Autodesk Inventor part; units mm, degrees
ref_plane "YZ Plane" through (0, 0, 0) normal (1, 0, 0) x (0, 1, 0)
ref_plane "XZ Plane" through (0, 0, 0) normal (0, 1, 0) x (-1, 0, 0)
ref_plane "XY Plane" through (0, 0, 0) normal (0, 0, 1) x (1, 0, 0)
sketch "Sketch1" plane through (0, 0, 0) normal (0, 0, 1) x (1, 0, 0)
  line L0 (-18.2, 27.5) -> (18.2, 27.5)
  line L1 (18.2, 27.5) -> (18.2, -27.5)
  line L2 (18.2, -27.5) -> (-18.2, -27.5)
  line L3 (-18.2, -27.5) -> (-18.2, 27.5)
  line L4 (0, -38.5) -> (0, 38.5)
  line L5 (-25.48, 0) -> (25.48, 0)
  circle A0 centre (-12.2, 21.5) radius 3
  circle A1 centre (-12.2, 21.5) radius 6 construction
  circle A2 centre (-12.2, -3.5) radius 3
  line L6 (-12.2, 27.5) -> (-12.2, -3.5) construction
  circle A3 centre (12.2, 21.5) radius 3
  circle A4 centre (12.2, -3.5) radius 3
  point P0 (0, 0)
  point P1 (0, 27.5)
  point P2 (-18.2, 0)
  dimension "d0" = 36.4
  dimension "d1" = 55
  dimension "d2" = 6
  dimension "d3" = 3
  dimension "d34" = 25
extrude "Extrusion1" add sketch "Sketch1" along normal blind 10
sketch "Sketch4" plane through (18.2, -27.5, 0) normal (1, 0, 0) x (0, 0, -1)
  circle A0 centre (-5, 17.5) radius 3 construction
  line L0 (-10, 55) -> (-10, 0)
  line L1 (-10, 27.5) -> (0, 27.5) construction
  line L2 (0, 55) -> (0, 0)
  circle A1 centre (-5, 37.5) radius 3
  line L3 (0, 0) -> (-10, 0)
  line L4 (-5, 0) -> (-5, 55) construction
  line L5 (0, 55) -> (-10, 55)
  circle A2 centre (-5, 17.5) radius 3.1
  dimension "d20" = 6
  dimension "d21" = 20
  dimension "d24" = 6.2
extrude "Extrusion4" cut sketch "Sketch4" against normal up to surface (36.4 mm away) contours A1 | A2
thread "Thread1"
sketch "Sketch5" plane through (18.2, -27.5, 0) normal (1, 0, 0) x (0, 0, -1)
  line L0 (-10, 55) -> (-10, 0)
  line L1 (0, -16.4451) -> (0, 0)
  line L2 (0, 0) -> (0, 55)
  line L3 (0, 0) -> (-10, 0)
  line L4 (0, -16.4451) -> (-10, 5)
  point P0 (0, 27.5)
  point P1 (-7.6685, 0)
  dimension "d30" = 5
  dimension "d31" = 25
extrude "Extrusion5" add sketch "Sketch5" against normal up to surface (36.4 mm away) contours L3 L1 L4
extrude "Extrusion6" cut sketch "Sketch5" against normal up to surface (36.4 mm away) contours L4 L3 L0
fillet "Fillet1" radius 1 5 edges at (0, 27.5, 0) (0, 27.5, 10) (0, -43.9451, 0) (18.2, -10, 8.1) (-18.2, -10, 8.1)
thread "Thread2"
thread "Thread3"
thread "Thread4"
thread "Thread5"
properties part number "Pedal Support 1"
Input: part model. Units: mm. Frame: model coordinates. Coordinates: 2 decimals unless noted, no trailing zeros. Loops run counter-clockwise (first coordinate to the right, second up) from the corner with the lowest first, then second, coordinate; pieces in that order, holes last. Notation, with made-up numbers: M 83.25,21.5 L 126.25,21.5 A18 ccw 126.25,37.5 Z; hole C 30.25,-38 d5. An arc over 180 degrees is marked long. Answer in a Markdown table with one row per item.
1. Section C-C, the plane x = -1. Output: boundary loops of the cut face in (y, z), then the cut area to 3 significant figures.
Response:
| item | result |
|---|---|
| outline | M -39.86,1.91 A1 ccw -39.43,0 L 26.5,0 A1 ccw 27.5,1 L 27.5,9 A1 ccw 26.5,10 L -22.5,10 Z; hole C -10,5 d6.2; hole C 10,5 d6 |
| area | 545 mm2 |
2. Section D-D, the plane z = 2.75. Count the separate pieces of the cut face and the enclosed holes in it, then the cut area to 3 significant figures.
Response:
| item | result |
|---|---|
| separate pieces | 3 |
| enclosed holes | 4 |
| area | 1,970 mm2 |
3. Section B-B, the plane y = -10. Output: boundary loops of the cut face in (x, z), then the cut area to 3 significant figures.
Response:
| item | result |
|---|---|
| outline | M -18.2,0 L 18.2,0 L 18.2,0.9 A1 ccw 17.2,1.9 L -17.2,1.9 A1 ccw -18.2,0.9 Z; M -18.2,9.1 A1 ccw -17.2,8.1 L 17.2,8.1 A1 ccw 18.2,9.1 L 18.2,10 L -18.2,10 Z |
| area | 137 mm2 |
4. Draft query along X for faces 1 (the cylindrical face through (-10.59, -6.03, 4.93)), 2 (the flat face through (0.255, -31.3, 5.896)), 3 (the flat face through (-18.2, -6, 3)). Return one class per face: pulls with the +X half, pulls with the -X half, needs draft (parallel to the pull), parting line crosses it, or undercut.
Response:
| item | result |
|---|---|
| face 1 | undercut |
| face 2 | needs draft |
| face 3 | pulls with the -X half |
5. Section A-A, the plane x = -12.2. Output: boundary loops of the cut face in (y, z), then the cut area to 3 significant figures.
Response:
| item | result |
|---|---|
| outline | M -39.86,1.91 A1 ccw -39.43,0 L -6.5,0 L -6.5,10 L -22.5,10 Z; M -0.5,0 L 18.5,0 L 18.5,10 L -0.5,10 Z; M 24.5,0 L 26.5,0 A1 ccw 27.5,1 L 27.5,9 A1 ccw 26.5,10 L 24.5,10 Z; hole C -10,5 d6.2; hole C 10,5 d6 |
| area | 425 mm2 |
6. First-contact query: pin 1 (3.5 mm diameter, centred on x = -12.2, y = 21.5, fed in from -Z); pin 2 (9.5 mm diameter, centred on x = -12.2, y = -3.5, fed in from -Z); pin 3 (3 mm diameter, centred on x = 13, z = 5.5, fed in from -Y). Flat tips, straight axial feed; report the tip coordinate or a pass-through.
Response:
| item | result |
|---|---|
| pin 1 | passes through |
| pin 2 | stops at z = 0 |
| pin 3 | stops at y = -35.37 |
7. Material intervals for line 1 (Y direction, x = -12.2, z = 5.5); line 2 (X direction, y = 21, z = 9.5); line 3 (Y direction, x = 12.2, z = 6.25), sorted ascending.
Response:
| item | result |
|---|---|
| line 1 | y = -32.15 to -13.06, -6.94 to -6.5, -0.5 to 7.04, 12.96 to 18.5, 24.5 to 27.5 |
| line 2 | x = -18.2 to -15.16, -9.24 to 9.24, 15.16 to 18.2 |
| line 3 | y = -30.54 to -12.84, -7.16 to -6.5, -0.5 to 7.27, 12.73 to 18.5, 24.5 to 27.5 |
